Check sheet for the drawn part. Datum: minimum x, y, z corner. Units: mm. A direction names the side the tool comes from. Round coordinates to 2 decimals unless told otherwise and drop trailing zeros. Order: outer loops, then holes, each group sorted by start corner. A loop starts at its lowest first (then second) coordinate and runs counter-clockwise, first axis right, second up.
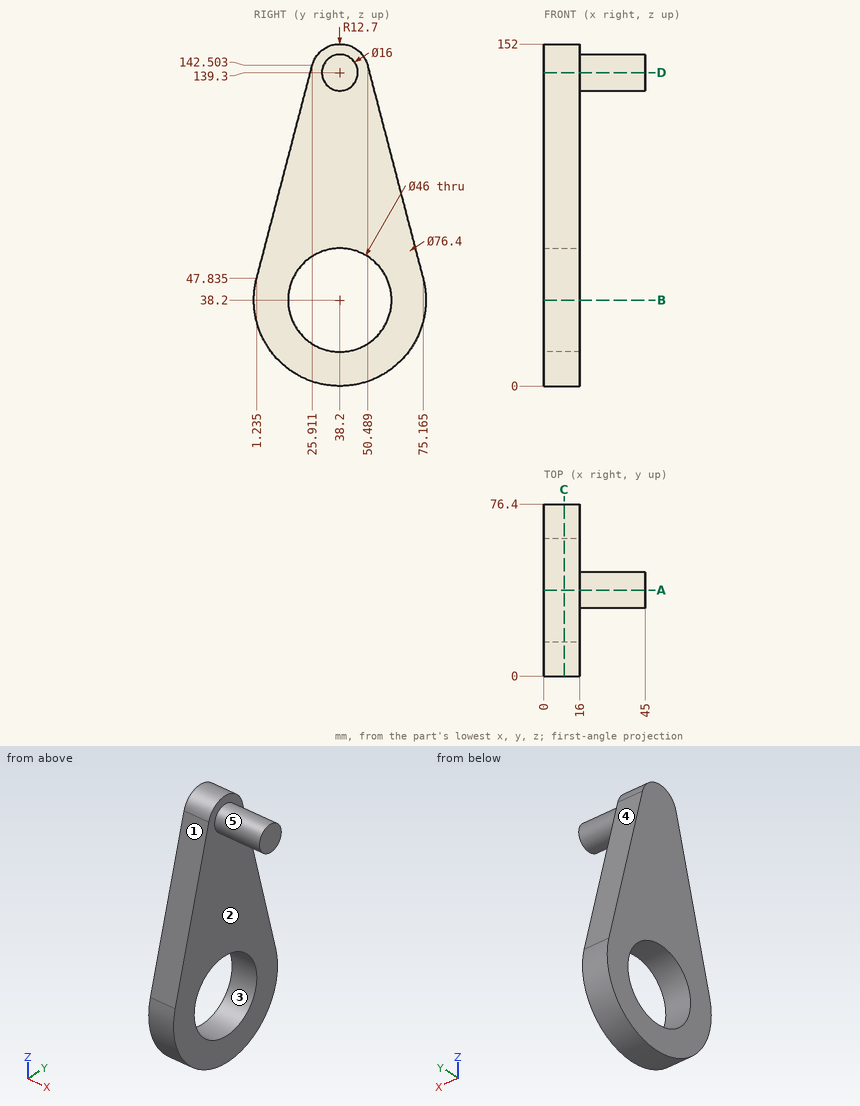
(1) Set-up check for the marked faces 4 and 5: record each of +Z, -Z, +X, -X, +Y, -Y from which the full face is reachable in a straight line by a thin tool's end or side.
Returned:
face 4: +Z, +X, -X, +Y
face 5: +X
(2) Sectioned sample at C-C, the plane x = 9. Record the cut outline in (y, z) (1 decimal).
Returned:
outline: (1.2, 47.8) arc R38.2 ccw (long way) to (75.2, 47.8) - (50.5, 142.5) arc R12.7 ccw to (25.9, 142.5) - close; hole circle Ø46 at (38.2, 38.2)
(3) Material ranges on line 1 (Y direction, x = 12, z = 38.2); line 2 (Z direction, x = 7, y = 38); line 3 (X direction, y = 57.5, z = 18.5), recorded low to high.
Returned:
line 1: y = 0 to 15.2, 61.2 to 76.4
line 2: z = 0 to 15.2, 61.2 to 152
line 3: x = 0 to 16
(4) Sectioned sample at B-B, the plane z = 38.2. Record the cut outline in (x, y).
Returned:
outline: (0, 0) - (16, 0) - (16, 15.2) - (0, 15.2) - close; (0, 61.2) - (16, 61.2) - (16, 76.4) - (0, 76.4) - close
(5) Sectioned sample at A-A, the plane y = 38.2. Record the cut outline in (x, z).
Returned:
outline: (0, 0) - (16, 0) - (16, 15.2) - (0, 15.2) - close; (0, 61.2) - (16, 61.2) - (16, 131.3) - (45, 131.3) - (45, 147.3) - (16, 147.3) - (16, 152) - (0, 152) - close
(6) Depth check by flat-ended pin: P1, Ø12, axis at x = 20, y = 44, coming from the +Z side; P2, Ø4, axis at y = 23.5, z = 112.5, coming from the +X side; P3, Ø5, axis at x = 14, z = 84.5, coming from the -Y side. Enter the tip coordinate at first touch or a pass-through.
Returned:
P1: stops at z = 151.93
P2: stops at x = 16
P3: stops at y = 10.14
(7) Sectioned sample at D-D, the plane z = 139.3. Record the cut outline in (x, y) (1 decimal).
Returned:
outline: (0, 25.1) - (16, 25.1) - (16, 30.2) - (45, 30.2) - (45, 46.2) - (16, 46.2) - (16, 51.3) - (0, 51.3) - close
(8) Draft check along Y on the marked faces 1, 2 and 3. Enter one of: released by +Y, released by -Y, zero draft, split by the parting line, or undercut.
Returned:
face 1: released by -Y
face 2: zero draft
face 3: undercut
